Geometry: final body of the model. Coordinates: model frame, mm. A direction names the side the tool comes from. Round coordinates to 2 decimals unless told otherwise and drop trailing zeros. Write each loop counter-clockwise with the first axis right and the second up, starting at its lowest first coordinate (ties: lowest second). Pieces come first, ordered by that corner, then holes. Notation, with made-up numbers: M 47.25,4 L 57.25,4 A19 ccw 57.25,26 Z; hole C 58.25,47.25 d7. An arc over 180 degrees is marked long. Put each result on its own line as item: value. Start each with the question number.
```python
from build123d import *

# Parameters (mm, degrees)
F1_DEPTH = 12.7
F3_DEPTH = 12.7
F5_DEPTH = 12.7


with BuildPart() as f1:
    # F0 (on Top) → F1 (new body)
    with BuildSketch(Plane.XY):
        Polygon((0, 762), (0, 0), (563.033164, 0), (563.033164, 598.91676), (413.93744, 625.206359), (38.1, 762), align=None)
    extrude(amount=F1_DEPTH)

    # F2 (on face) → F3 (join)
    with BuildSketch(Plane.XY.offset(12.7)):
        Polygon((371.488792, 559.833981), (25.4, 685.8), (12.369033, 649.997711), (358.457825, 524.031692), align=None)
    extrude(amount=F3_DEPTH)

    # F4 (on face) → F5 (join)
    with BuildSketch(Plane(origin=(0, 0, 0), x_dir=(1, 0, 0), z_dir=(0, 0, -1))):
        Polygon((12.369033, -649.997711), (25.4, -685.8), (371.488792, -559.833981), (358.457825, -524.031692), align=None)
    extrude(amount=F5_DEPTH)


solid = f1.part
```
1) Access query for faces 1 (the face through (182.991, 587.896, 18.961)), 2 (the face through (200.867, 621.935, 18.961)), 3 (the face through (187.84, 586.13, -6.26)), 4 (the face through (196.02, 623.7, -6.26)). Directions: +Z, -Z, +X, -X, +Y, -Y. A direction counts if a zero-diameter tool reaches every point of the face in a straight line with its end or side. Return the directions, or none.
2) First-contact query: pin 1 (1.5 mm diameter, centred on x = 81, z = 2, fed in from +Y); pin 2 (3 mm diameter, centred on y = 584, z = 11.5, fed in from -X); pin 3 (3 mm diameter, centred on x = 314, z = 7, fed in from +Y); pin 4 (1.5 mm diameter, centred on x = 504.5, z = 2.5, fed in from +Y). Flat tips, straight axial feed; report the tip coordinate or a pass-through.
3) Section D-D, the plane x = 459. Output: boundary loops of the cut face in (y, z).
4) Ray query, probe 1 along Z at (x, y) = (238.5, 643); probe 2 along Y at (x, z) = (345.5, 1); probe 3 along Y at (x, z) = (127.5, -7.5). Return the intervals inside material, ascending.
5) Section B-B, the plane y = 637. Output: boundary loops of the cut face in (x, z).
6) Section C-C, the plane y = 359. Output: boundary loops of the cut face in (x, z).
7) Section A-A, the plane x = 128.5. Output: boundary loops of the cut face in (y, z), and give its area (3 significant figures).
Solved:
1. face 1: +Z, -X, -Y
1. face 2: +Z, +X, +Y
1. face 3: -Z, -X, -Y
1. face 4: -Z, +X, +Y
2. pin 1: stops at y = 746.66
2. pin 2: stops at x = 0
2. pin 3: stops at y = 662.13
2. pin 4: stops at y = 609.37
3. outline: M 0,0 L 617.26,0 L 617.26,12.7 L 0,12.7 Z
4. probe 1: z = 0 to 12.7
4. probe 2: y = 0 to 650.12
4. probe 3: y = 608.09 to 648.64
5. outline: M 0,0 L 48.08,0 L 48.08,-12.7 L 159.48,-12.7 L 159.48,0 L 381.53,0 L 381.53,12.7 L 159.48,12.7 L 159.48,25.4 L 48.08,25.4 L 48.08,12.7 L 0,12.7 Z
6. outline: M 0,0 L 563.03,0 L 563.03,12.7 L 0,12.7 Z
7. outline: M 0,0 L 607.73,0 L 607.73,-12.7 L 648.27,-12.7 L 648.27,0 L 729.1,0 L 729.1,12.7 L 648.27,12.7 L 648.27,25.4 L 607.73,25.4 L 607.73,12.7 L 0,12.7 Z
7. area: 10,300 mm2
